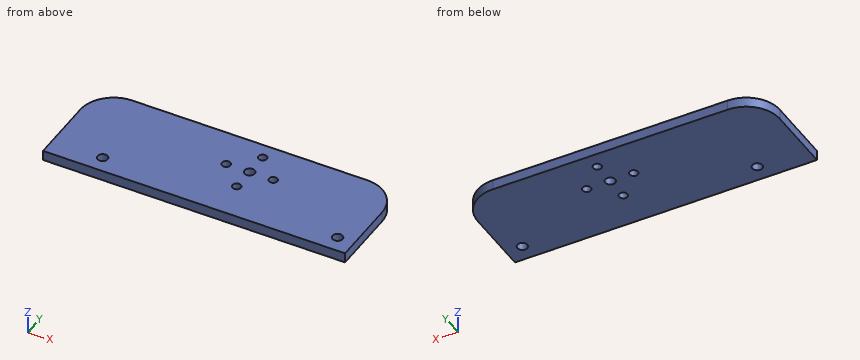
```python
from build123d import *

# Parameters (mm, degrees)
SKETCH_1_W          = 90
SKETCH_1_H          = 30
EXTRUDE_1_DEPTH     = 3
SKETCH_3_R          = 1.5
SKETCH_3_R_2        = 1.25
CUT_EXTRUDE_2_DEPTH = 10
SKETCH_4_R          = 1.5
CUT_EXTRUDE_3_DEPTH = 10
FILLET_1_R          = 10


with BuildPart() as part:
    # 草图1 → 凸台-拉伸1 (new body)
    with BuildSketch(Plane.XY):
        Rectangle(SKETCH_1_W, SKETCH_1_H)
    extrude(amount=EXTRUDE_1_DEPTH)

    # 草图3 → 切除-拉伸2 (cut)
    with BuildSketch(Plane(origin=(0, 0, 0), x_dir=(-1, 0, 0), z_dir=(0, 0, -1))):
        with Locations((-6.49227102, 3.236967106)):
            Circle(SKETCH_3_R)
        with Locations((-13.49227102, 3.236967106)):
            Circle(SKETCH_3_R_2)
        with Locations((-6.49227102, 10.236967106)):
            Circle(SKETCH_3_R_2)
        with Locations((-6.49227102, -3.763032894)):
            Circle(SKETCH_3_R_2)
        with Locations((0.50772898, 3.236967106)):
            Circle(SKETCH_3_R_2)
    extrude(amount=-CUT_EXTRUDE_2_DEPTH, mode=Mode.SUBTRACT)

    # 草图4 → 切除-拉伸3 (cut)
    with BuildSketch(Plane(origin=(0, 0, 0), x_dir=(-1, 0, 0), z_dir=(0, 0, -1))):
        with Locations((-40, -10)):
            Circle(SKETCH_4_R)
        with Locations((30, -10)):
            Circle(SKETCH_4_R)
    extrude(amount=-CUT_EXTRUDE_3_DEPTH, mode=Mode.SUBTRACT)

    # 圆角1
    fillet_1_edges = [part.edges().sort_by_distance(p)[0] for p in [
        (-45, 15, 1.5),
        (45, 15, 1.5),
    ]]
    fillet(fillet_1_edges, radius=FILLET_1_R)


solid = part.part
```
Geometry: final body of the model. Coordinates: model frame, mm. Coordinates: 2 decimals unless noted, no trailing zeros. Write each loop counter-clockwise with the first axis right and the second up, starting at its lowest first coordinate (ties: lowest second). Pieces come first, ordered by that corner, then holes. Notation, with made-up numbers: M 38.5,-10 L 46.5,-10 A28 cw 46.5,13 Z; hole C -24.75,34.25 d6. An arc over 180 degrees is marked long. Answer as CSV lines item,"result". Start each with the question number.
Q1. Cut plane B-B on x = -30. Return the cut outline in (y, z).
Q2. Pin query (flat end, axial travel): P1, Ø2.5, axis at x = -30, y = -10, coming from the -Z side; P2, Ø1, axis at y = 7, z = 2, coming from the -X side. Return the tip coordinate at first contact, or that it passes through.
Q3. Cut plane D-D on x = 40. Return the cut outline in (y, z), then the cut area to 3 significant figures.
Q4. Cut plane C-C on z = 2.5. Return the cut outline in (x, y).
Q5. Line query: line 1 (Y direction, x = -30, z = 1.1); line 2 (X direction, y = 4, z = 1.7); line 3 (Y direction, x = 40, z = 1.8). Output: solid intervals per line, ascending. Write a range as from..to.
Q6. Cut plane A-A on y = -10. Return the cut outline in (x, z).
Findings below:
1,outline,"M -15,0 L -11.5,0 L -11.5,3 L -15,3 Z; M -8.5,0 L 15,0 L 15,3 L -8.5,3 Z"
2,P1,"passes through"
2,P2,"stops at x = -44.89"
3,outline,"M -15,0 L -11.5,0 L -11.5,3 L -15,3 Z; M -8.5,0 L 13.66,0 L 13.66,3 L -8.5,3 Z"
3,area,"77.0 mm2"
4,outline,"M -45,-15 L 45,-15 L 45,5 A10 ccw 35,15 L -35,15 A10 ccw -45,5 Z; hole C -30,-10 d3; hole C -0.51,3.24 d2.5; hole C 6.49,3.24 d3; hole C 6.49,-3.76 d2.5; hole C 6.49,10.24 d2.5; hole C 13.49,3.24 d2.5; hole C 40,-10 d3"
5,line 1,"y = -15..-11.5, -8.5..15"
5,line 2,"x = -45..-1.5, 0.48..5.2, 7.78..12.5, 14.48..45"
5,line 3,"y = -15..-11.5, -8.5..13.66"
6,outline,"M -45,0 L -31.5,0 L -31.5,3 L -45,3 Z; M -28.5,0 L 38.5,0 L 38.5,3 L -28.5,3 Z; M 41.5,0 L 45,0 L 45,3 L 41.5,3 Z"
